Source: three-view drawing plus pictorial views. Frame: mm from the lowest corner of the part. A direction names the side the tool comes from. Coordinates: 2 decimals unless noted, no trailing zeros. Write each loop counter-clockwise with the first axis right and the second up, starting at its lowest first coordinate (ties: lowest second). Pieces come first, ordered by that corner, then holes. Notation, with made-up numbers: (43.5, 57.25) - (101.5, 57.25) arc R21 cw to (101.5, 95.25) - close; hole circle Ø4 at (-17.5, 48). An arc over 180 degrees is marked (long way). One line per item, written item: value.
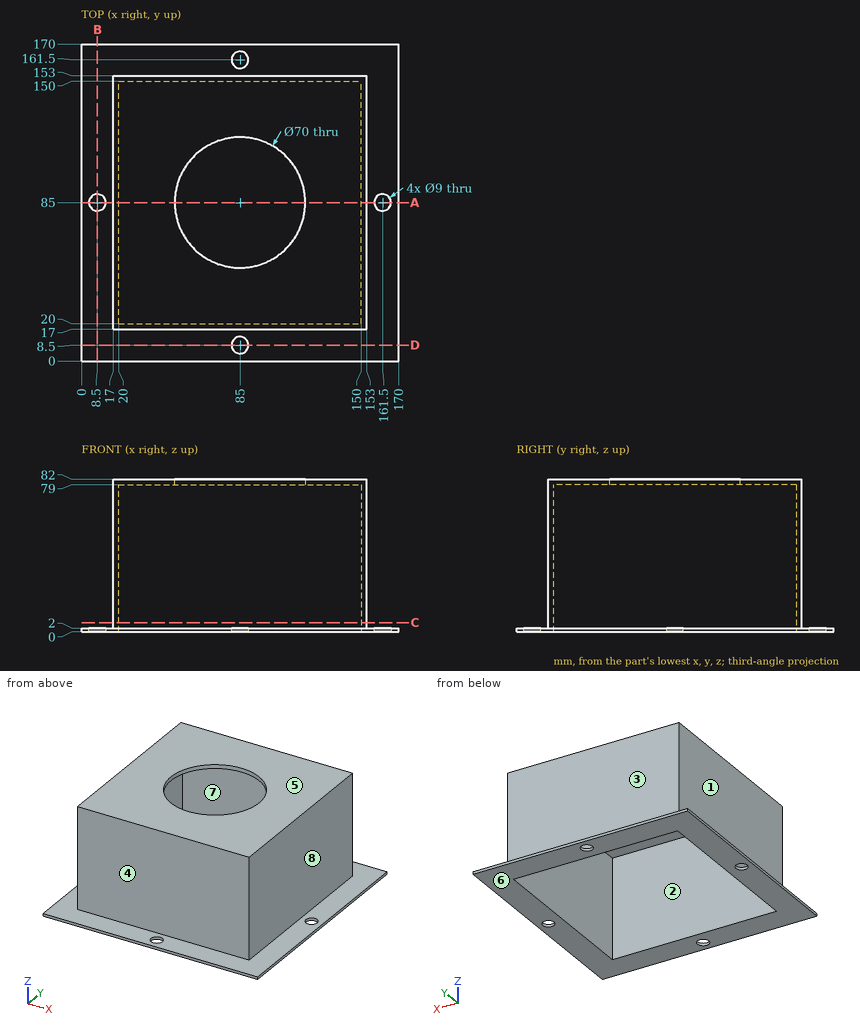
1) Section query A-A on y = 85. Output: boundary loops of the cut face in (x, z).
Values found:
outline: (0, 0) - (4, 0) - (4, 2) - (0, 2) - close; (13, 0) - (20, 0) - (20, 79) - (50, 79) - (50, 82) - (17, 82) - (17, 2) - (13, 2) - close; (120, 79) - (150, 79) - (150, 0) - (157, 0) - (157, 2) - (153, 2) - (153, 82) - (120, 82) - close; (166, 0) - (170, 0) - (170, 2) - (166, 2) - close
2) Contact query for flat-ended pins moving along their axis: P1, Ø14.5, axis at x = 85, y = 8.5, coming from the -Z side; P2, Ø1.5, axis at x = 44, y = 140.5, coming from the -Z side; P3, Ø6, axis at x = 52, z = 29.5, coming from the -Y side; P4, Ø12, axis at x = 103, z = 48, coming from the +Y side. Output: stop coordinate, or through.
Values found:
P1: z = 0
P2: z = 79
P3: y = 17
P4: y = 153
3) Section query B-B on x = 8.5. Output: boundary loops of the cut face in (y, z).
Values found:
outline: (0, 0) - (80.5, 0) - (80.5, 2) - (0, 2) - close; (89.5, 0) - (170, 0) - (170, 2) - (89.5, 2) - close
4) Draft query along X for the marked faces 6, 7 and 8. Return one class per face: released by +X, released by -X, zero draft, split by the parting line, or undercut.
Values found:
face 6: zero draft
face 7: undercut
face 8: released by +X
5) Section query C-C on z = 5. Output: boundary loops of the cut face in (x, y), then the cut area to 3 significant figures.
Values found:
outline: (17, 17) - (153, 17) - (153, 153) - (17, 153) - close; hole (20, 20) - (150, 20) - (150, 150) - (20, 150) - close
area: 1,600 mm2
6) Reachability of the marked faces 1, 2, 3, 4 and 5 from +Z, -Z, +X, -X, +Y, -Y: full face, straight path, thin tool, end or side. Return the list, or none.
Values found:
face 1: +Z, -X, +Y, -Y
face 2: -Z
face 3: +Z, +X, -X, +Y
face 4: +Z, +X, -X, -Y
face 5: +Z, +X, -X, +Y, -Y
7) Material intervals for line 1 (Y direction, x = 85, z = 1.2); line 2 (Y direction, x = 57, z = 68), sorted ascending.
Values found:
line 1: 0 to 4, 13 to 20, 150 to 157, 166 to 170
line 2: 17 to 20, 150 to 153
